The listing builds one solid part. Answer for the finished solid, in the listing's coordinates (mm). Face numbers are marked on the shaded views. A direction names the side the tool comes from. Give positions to 0.01 mm unless a question says otherwise; leave off trailing zeros. Loops run counter-clockwise (first coordinate to the right, second up) from the corner with the lowest first, then second, coordinate; pieces in that order, holes last. Notation, with made-up numbers: M 22,54.5 L 73,54.5 A21 ccw 73,67.5 Z; hole C -12.5,30 d9. An arc over 180 degrees is marked long. One line per item, written item: value. Start each with the question number.
Q1. A cutting plane is placed at D-D, the plane z = 25.9. Determine the outline of the cut face in (x, y).
Q2. Consider L1, parallel to Z at x = 64, y = 8.5; L2, parallel to X at y = 2.25, z = 13; L3, parallel to Y at x = 78, z = 11. Determine where each line is inside the solid, lowest interval first.
Q3. A cutting plane is placed at A-A, the plane z = 4. Determine the outline of the cut face in (x, y).
Q4. The mould has two halves that part along Z. Classify the marked faces 1, 2 and 3: +Z half, -Z half, draft (parallel to the pull), parting line (faces both ways), or undercut.
Q5. Flat-ended cylindrical pins translate along their axes: pin 1 (1 mm diameter, centred on y = 20.5, z = 37.5, fed in from +X); pin 2 (1.5 mm diameter, centred on y = 8, z = 38, fed in from +X); pin 3 (4 mm diameter, centred on x = 81.4, z = 30.9, fed in from -Y). Find the tip coordinate at first contact, or state that the pin passes through.
Q6. For the marked faces 4, 5 and 6, determine the directions among +Z, -Z, +X, -X, +Y, -Y from which every point of the face is accessible in a straight line to the end or side of a thin tool.
Q7. A cutting plane is placed at B-B, the plane x = 81.4. State how many separate pieces and enclosed holes the cut face has, and give its area (3 significant figures).
Q8. A cutting plane is placed at C-C, the plane x = 29.5. Determine the outline of the cut face in (y, z).
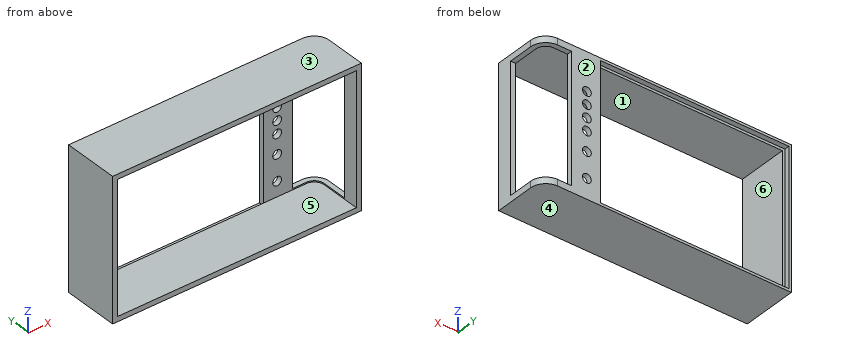
Autodesk Fusion 360 part; units mm, degrees
sketch "Boceto1" plane through (0, 0, 0) normal (0, 0, 1) x (1, 0, 0)
  line L0 (0, 0) -> (99, 0)
  line L1 (99, 0) -> (99, 22)
  line L2 (99, 22) -> (0, 22)
  line L3 (0, 22) -> (0, 0)
  dimension "d1" = 22
  dimension "d2" = 99
extrude "Extruir1" add sketch "Boceto1" along normal blind 56
shell "Vaciado1" thickness 2 removed faces 1 at (33, 0, 18.6667)
sketch "Boceto2" plane through (0, 22, 0) normal (0, 1, 0) x (-1, 0, 0)
  line L0 (-99, 0) -> (0, 0)
  line L1 (0, 0) -> (0, 56)
  line L2 (0, 56) -> (-99, 56)
  line L3 (-99, 56) -> (-99, 0)
  line L4 (-1, 1) -> (-76, 1)
  line L5 (-76, 1) -> (-76, 55)
  line L6 (-76, 55) -> (-1, 55)
  line L7 (-1, 55) -> (-1, 1)
  dimension "d6" = 1
  dimension "d7" = 1
  dimension "d8" = 1
  dimension "d9" = 75
extrude "Extruir2" cut sketch "Boceto2" against normal blind 2 contours L4 L5 L6 L7
sketch "Boceto3" plane through (0, 22, 0) normal (0, 1, 0) x (-1, 0, 0)
  line L0 (-76, 1) -> (-76, 55)
  line L1 (-76, 55) -> (-1, 55)
  line L2 (-1, 55) -> (-1, 1)
  line L3 (-1, 1) -> (-76, 1)
  line L4 (-99, 0) -> (0, 0)
  line L5 (0, 0) -> (0, 56)
  line L6 (0, 56) -> (-99, 56)
  line L7 (-99, 56) -> (-99, 0)
  line L8 (-99, 2.5) -> (-87.5, 2.5)
  line L9 (-87.5, 2.5) -> (-87.5, 53.5)
  line L10 (-87.5, 53.5) -> (-99, 53.5)
  line L11 (-99, 53.5) -> (-99, 2.5)
  circle A0 centre (-81.4, 40.9) radius 1.75
  circle A1 centre (-81.4, 18.1) radius 1.75
  circle A2 centre (-81.4, 7.94) radius 1.75
  circle A3 centre (-81.4, 35.9) radius 1.75
  circle A4 centre (-81.4, 30.9) radius 1.75
  circle A5 centre (-81.4, 25.9) radius 1.75
  dimension "d12" = 2.5
  dimension "d13" = 2.5
  dimension "d14" = 11.5
  dimension "d29" = 0
  dimension "d30" = -15
  dimension "d31" = 6.1
  dimension "d32" = 3.5
  dimension "d33" = 3.5
  dimension "d34" = 3.5
  dimension "d35" = 10.16
  dimension "d36" = 12.6
  dimension "d37" = 7.8
extrude "Extruir3" cut sketch "Boceto3" against normal blind 16 contours L7 L8 L9 L10 L11 | A0 | A1 | A2 | A3 | A4 | A5
fillet "Empalme1" radius 6 2 edges at (99, 22, 1.25) (99, 22, 54.75)
fillet "Empalme1" radius 4 2 edges at (97, 20, 2.25) (97, 20, 53.75)
equation "d35 = ( 4 * 2.54 ) * 1 mm"
Answer block:
1. outline: M 0,0 L 2,0 L 2,20 L 1,20 L 1,22 L 0,22 Z; M 76,20 L 79.65,20 L 79.65,22 L 76,22 Z; M 83.15,20 L 87.5,20 L 87.5,22 L 83.15,22 Z; M 97,0 L 99,0 L 99,6 L 97,6 Z
2. L1: 0 to 2, 54 to 56
2. L2: 0 to 2, 97 to 99
2. L3: 20 to 22
3. outline: M 0,0 L 2,0 L 2,20 L 1,20 L 1,22 L 0,22 Z; M 76,20 L 87.5,20 L 87.5,22 L 76,22 Z; M 97,0 L 99,0 L 99,6 L 97,6 Z
4. face 1: undercut
4. face 2: draft
4. face 3: +Z half
5. pin 1: x = 87.5
5. pin 2: x = 2
5. pin 3: y = 20
6. face 4: -Z, +X, -X, +Y, -Y
6. face 5: -Y
6. face 6: +Y, -Y
7. separate pieces: 7
7. enclosed holes: 0
7. area: 150 mm^2
8. outline: M 0,0 L 22,0 L 22,1 L 20,1 L 20,2 L 0,2 Z; M 0,54 L 20,54 L 20,55 L 22,55 L 22,56 L 0,56 Z
